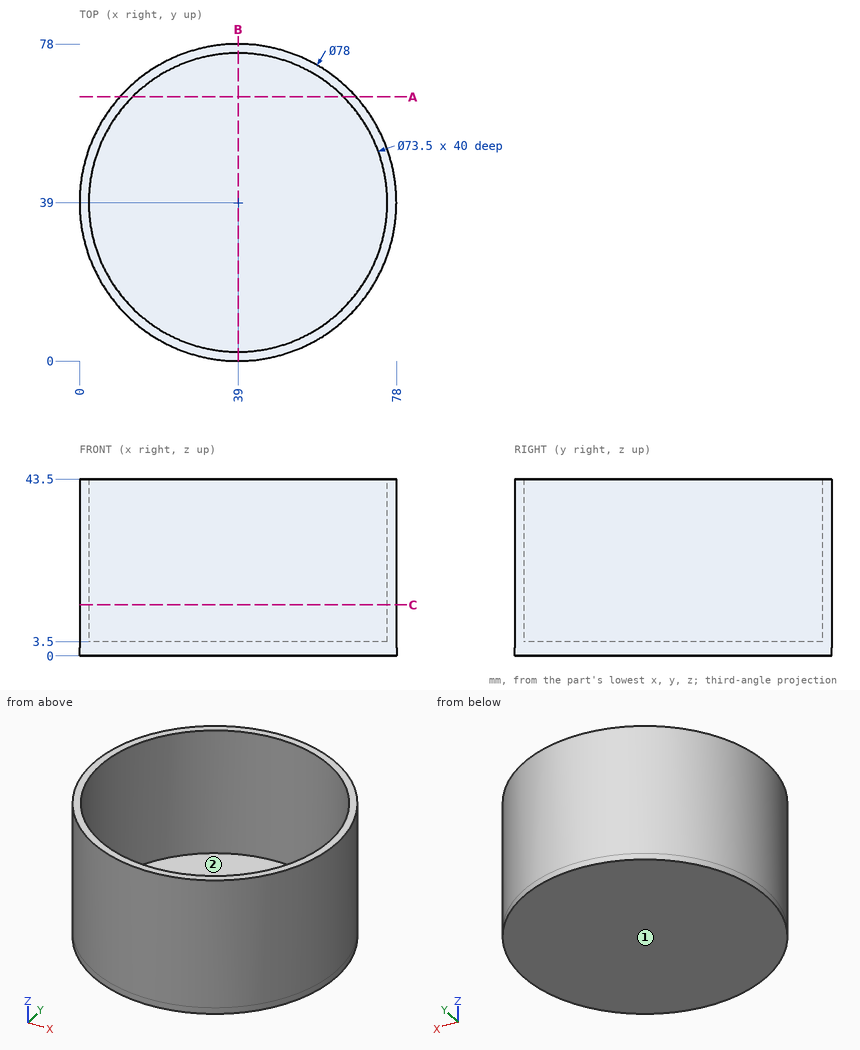
The figure shows three views and two pictorial views of one solid part (mm, origin at its lowest corner). Answer the questions. Coordinates: 2 decimals unless noted, no trailing zeros. Loops run counter-clockwise (first coordinate to the right, second up) from the corner with the lowest first, then second, coordinate; pieces in that order, holes last. Notation, with made-up numbers: (0, 12.5) -> (43, 12.5) arc R22 cw to (43, 25.5) -> close; hole circle Ø6 at (-3, -1). An arc over 180 degrees is marked (long way). Return JSON: item names as keys, results as strings. Group by question number.
(1) A cutting plane is placed at C-C on z = 12.5. Write down the section's boundary in (x, y), and give its area (3 significant figures).
(2) A cutting plane is placed at A-A on y = 65. Write down the section's boundary in (x, z), and give its area (3 significant figures).
(3) Determine the mould class of the marked faces 1 and 2 for opening direction X: released by +X, released by -X, zero draft, split by the parting line, or undercut.
(4) A cutting plane is placed at B-B on x = 39. Write down the section's boundary in (y, z), and give its area (3 significant figures).
(5) Find the intervals of material crossed by probe 1 along Y at (x, z) = (39, 33.5); probe 2 along Z at (x, y) = (17, 12); probe 3 along Y at (x, z) = (27.5, 20), in increasing order. Write a range as from..to.
(6) Given pin 1 Ø12 at (x, y) = (31.5, 55.5) entering from +Z; pin 2 Ø5 at (y, z) = (50.5, 31.5) entering from -X; pin 3 Ø8 at (x, z) = (22.5, 10.5) entering from -Y; pin 4 Ø4 at (x, y) = (10.5, 10.5) entering from -Z, each flat-ended and moving along its own axis, determine where each tip first touches the part or whether it passes through.
The answers:
{
 "1": {"outline": "circle Ø78 at (39, 39); hole circle Ø73.5 at (39, 39)", "area": "535 mm^2"},
 "2": {"outline": "(9.93, 0) -> (68.07, 0) -> (68.07, 43.5) -> (64.97, 43.5) -> (64.97, 3.5) -> (13.03, 3.5) -> (13.03, 43.5) -> (9.93, 43.5) -> close", "area": "451 mm^2"},
 "3": {"face 1": "zero draft", "face 2": "undercut"},
 "4": {"outline": "(0, 0) -> (78, 0) -> (78, 43.5) -> (75.75, 43.5) -> (75.75, 3.5) -> (2.25, 3.5) -> (2.25, 43.5) -> (0, 43.5) -> close", "area": "453 mm^2"},
 "5": {"probe 1": "y = 0..2.25, 75.75..78", "probe 2": "z = 0..3.5", "probe 3": "y = 1.73..4.1, 73.9..76.27"},
 "6": {"pin 1": "stops at z = 3.5", "pin 2": "stops at x = 1.05", "pin 3": "stops at y = 2.06", "pin 4": "stops at z = 0"}
}
